Input: dimensioned drawing with shaded views. Units: mm. Origin: part minimum x, y, z. Coordinates: 2 decimals unless noted, no trailing zeros. Order: outer loops, then holes, each group sorted by start corner. A loop starts at its lowest first (then second) coordinate and runs counter-clockwise, first axis right, second up. Notation, with made-up numbers: (34.25, 68.5) - (83.25, 68.5) arc R7 cw to (83.25, 72.5) - close; hole circle Ø3 at (55, 73.5). An arc over 180 degrees is marked (long way). One line per question, with ' | ' between items. Start each with the question number.
(1) Contact query for flat-ended pins moving along their axis: P1, Ø5.5, axis at y = 168.5, z = 29, coming from the -X side; P2, Ø4, axis at x = 101, z = 31.5, coming from the -Y side; P3, Ø4, axis at x = 183.5, z = 18.5, coming from the +Y side. Output: stop coordinate, or through.
(2) Section B-B (x = 144). Return the cut outline in (y, z), then the cut area to 3 significant figures.
(3) Draft query along Y for the marked faces 1, 2 and 3. Return one class per face: +Y half, -Y half, draft (parallel to the pull), parting line (faces both ways), or undercut.
(4) Section D-D (y = 264). Return the cut outline in (x, z).
(5) Line query: line 1 along Y through (x, z) = (144, 22); line 2 along X through (y, z) = (133.5, 15) (1 decimal); line 3 along X through (y, z) = (126.5, 17) (1 decimal). Output: solid intervals per line, ascending.
(6) Section C-C (z = 17). Return the cut outline in (x, y), then the cut area to 3 significant figures.
(7) Section A-A (y = 144). Return the cut outline in (x, z), then the cut area to 3 significant figures.
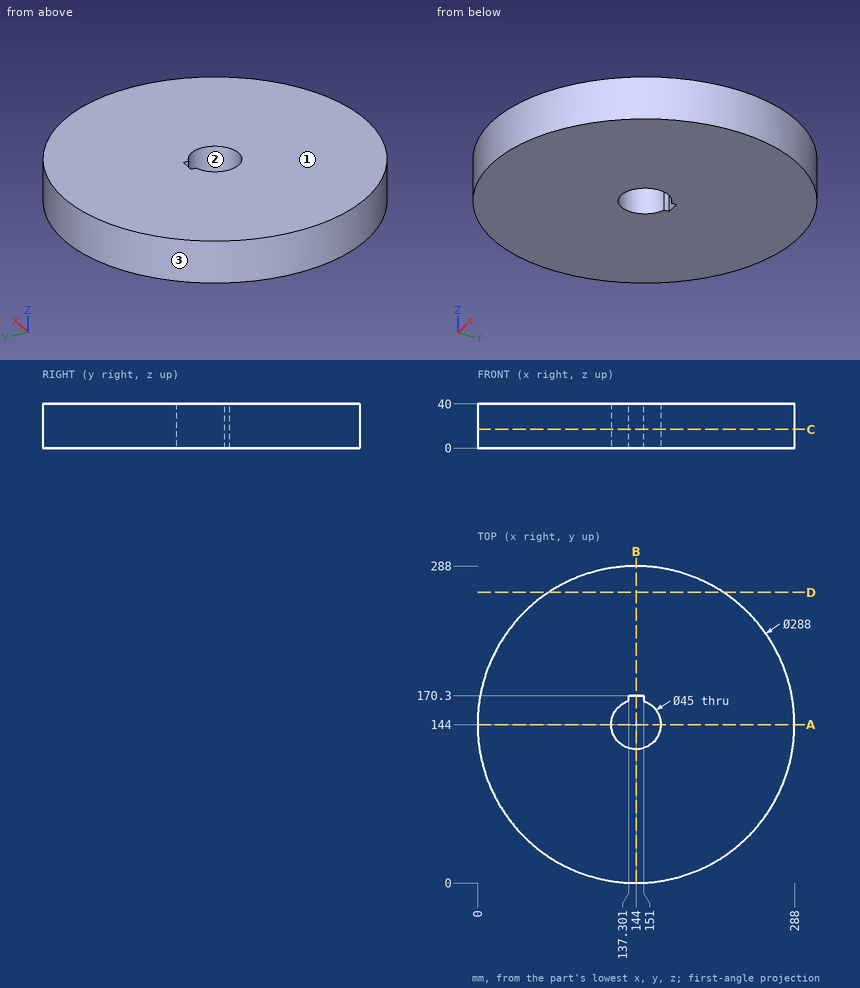
Response values:
1) P1: stops at x = 1.65 | P2: stops at y = 5.96 | P3: stops at y = 283.03
2) outline: (0, 0) - (121.5, 0) - (121.5, 40) - (0, 40) - close; (170.3, 0) - (288, 0) - (288, 40) - (170.3, 40) - close | area: 9,570 mm²
3) face 1: draft | face 2: undercut | face 3: parting line
4) outline: (64.4, 0) - (223.6, 0) - (223.6, 40) - (64.4, 40) - close
5) line 1: y = 0 to 121.5, 170.3 to 288 | line 2: x = 0.4 to 124.1, 163.9 to 287.6 | line 3: x = 1.1 to 129.9, 158.1 to 286.9
6) outline: circle Ø288 at (144, 144); hole (137.3, 165.48) arc R22.5 ccw (long way) to (151, 165.38) - (151, 170.3) - (137.3, 170.3) - close | area: 63,500 mm²
7) outline: (0, 0) - (121.5, 0) - (121.5, 40) - (0, 40) - close; (166.5, 0) - (288, 0) - (288, 40) - (166.5, 40) - close | area: 9,720 mm²
